Geometry: final body of the model. Coordinates: model frame, mm. Face numbers are marked on the shaded views. A direction names the side the tool comes from. Coordinates: 2 decimals unless noted, no trailing zeros. Order: outer loops, then holes, each group sorted by start corner. A loop starts at its lowest first (then second) coordinate and runs counter-clockwise, first axis right, second up. Notation, with made-up numbers: M 53.5,-8 L 109.5,-8 A15 cw 109.5,13 Z; hole C 77.5,-4 d1. An arc over 180 degrees is marked long. Write item = value, one per line.
from build123d import *

# Parameters (mm, degrees)
F1_DEPTH  = 320
F2_W      = 30
F2_H      = 320
F3_DEPTH  = 428
F5_DEPTH  = 205
F7_W      = 260
F7_H      = 128.6325914682
F8_DEPTH  = 30
F9_W      = 7.5
F9_H      = 457.219858036
F10_DEPTH = 977
F6_W      = 20
F6_H      = 50
F6_H_2    = 25
F11_DEPTH = 25
F12_R     = 5.1978686685
F13_DEPTH = 63


with BuildPart() as f1:
    # F0 (on Front) → F1 (new body)
    with BuildSketch(Plane.XZ):
        with BuildLine():
            Line((150.299176857, 1.1440683747), (180.299176857, 1.1440683747))
            Line((180.299176857, 1.1440683747), (340.299176857, 1.1440683747))
            add(Edge.make_bspline(
                [(340.299176857, 1.1440683747), (349.1569172885, 24.1151609846), (251.1032390966, 88.0444564268), (175.3079980464, 151.1440683747)],
                knots=[0.4586039165, 0.4586039165, 0.4586039165, 0.4586039165, 1, 1, 1, 1], degree=3))
            Line((175.3079980464, 151.1440683747), (145.3079980464, 151.1440683747))
            Line((145.3079980464, 151.1440683747), (0.299176857, 1.1440683747))
            Line((0.299176857, 1.1440683747), (100.299176857, 1.1440683747))
            Line((100.299176857, 1.1440683747), (150.299176857, 1.1440683747))
        make_face()
    extrude(amount=F1_DEPTH)

    # F2 (on face) → F3 (join)
    with BuildSketch(Plane.XY.offset(151.1440683747)):
        with Locations((160.3079980464, -160)):
            Rectangle(F2_W, F2_H)
    extrude(amount=F3_DEPTH)

    # F4 (on face) → F5 (cut)
    with BuildSketch(Plane(origin=(145.3079980464, 0, 0), x_dir=(0, -1, 0), z_dir=(-1, 0, 0))):
        with BuildLine():
            Line((0, 579.1440683747), (0, 151.1440683747))
            add(Edge.make_bspline(
                [(60, 368.6685562134), (50.1739969339, 296.0916949665), (25.086998467, 223.6178816706), (0, 151.1440683747)],
                knots=[0.4913001533, 0.4913001533, 0.4913001533, 0.4913001533, 1, 1, 1, 1], degree=3))
            Line((60, 368.6685562134), (60, 579.1440683747))
            Line((60, 579.1440683747), (0, 579.1440683747))
        make_face()
        with BuildLine():
            add(Edge.make_bspline(
                [(320, 151.1440683747), (294.913001533, 223.6178816706), (269.8260030661, 296.0916949665), (260, 368.6685562134)],
                knots=[0, 0, 0, 0, 0.5086998467, 0.5086998467, 0.5086998467, 0.5086998467], degree=3))
            Line((320, 151.1440683747), (320, 579.1440683747))
            Line((320, 579.1440683747), (260, 579.1440683747))
            Line((260, 579.1440683747), (260, 368.6685562134))
        make_face()
    extrude(amount=-F5_DEPTH, mode=Mode.SUBTRACT)

    # F7 (on face) → F8 (cut)
    with BuildSketch(Plane(origin=(-0.4170581217, 0, 0.4031807106), x_dir=(0, -1, 0), z_dir=(-0.7189672474, 0, 0.6950439534))):
        with Locations((160, 105.3467844897)):
            Rectangle(F7_W, F7_H)
    extrude(amount=-F8_DEPTH, mode=Mode.SUBTRACT)

    # F9 (on face) → F10 (cut)
    with BuildSketch(Plane.XZ.offset(320)):
        with Locations((154.0579980464, 379.7539973927)):
            Rectangle(F9_W, F9_H)
        with Locations((166.5579980464, 379.7539973927)):
            Rectangle(F9_W, F9_H)
    extrude(amount=-F10_DEPTH, mode=Mode.SUBTRACT)

    # F6 (on face) → F11 (join)
    with BuildSketch(Plane.YZ.offset(175.3079980464)):
        with Locations((-250, 554.1440683747)):
            Rectangle(F6_W, F6_H)
        with Locations((-70, 554.1440683747)):
            Rectangle(F6_W, F6_H)
        with Locations((-230, 406.1685562134)):
            Rectangle(F6_W, F6_H_2)
        with Locations((-90, 406.1685562134)):
            Rectangle(F6_W, F6_H_2)
    extrude(amount=-F11_DEPTH)

    # F12 (on Right) → F13 (cut)
    with BuildSketch(Plane.YZ):
        with Locations((-268.3978974819, 7.7915792353)):
            Circle(F12_R)
    extrude(amount=F13_DEPTH, mode=Mode.SUBTRACT)


solid = f1.part
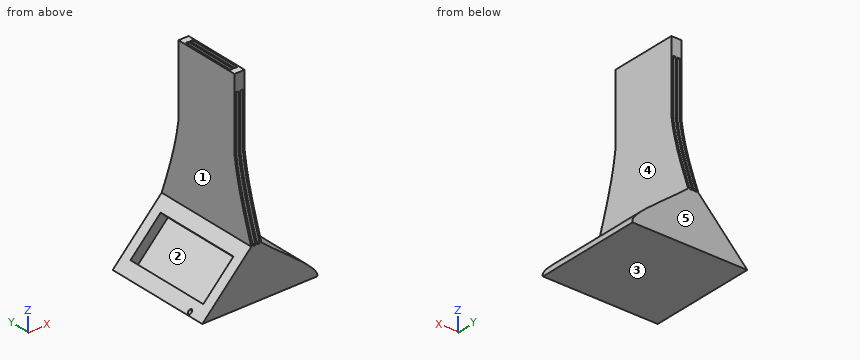
1) Section C-C, the plane y = -231.5. Give the number of separate pieces and of enclosed holes in the cut face, and give its area (3 significant figures).
Numbers:
separate_pieces = 1
enclosed_holes = 2
area = 32,200 mm²
2) Section A-A, the plane z = 539. Return loops of the section in (x, y).
Numbers:
outline = M 145.31,-260 L 175.31,-260 L 175.31,-60 L 145.31,-60 Z; hole M 150.31,-240 L 157.81,-240 L 157.81,-80 L 150.31,-80 Z; hole M 162.81,-240 L 170.31,-240 L 170.31,-80 L 162.81,-80 Z
3) Mould query, pull axis Z, two halves, no side actions, for the marked faces 1, 2 and 3. Classes: pulls with the +Z half, pulls with the -Z half, needs draft (parallel to the pull), parting line crosses it, or undercut.
Numbers:
face_1 = needs draft
face_2 = undercut
face_3 = pulls with the -Z half
4) Pin query (flat end, axial travel): pin 1 (8 mm diameter, centred on x = 156, z = 404, fed in from -Y); pin 2 (5 mm diameter, centred on y = -111, z = 424, fed in from -X); pin 3 (5 mm diameter, centred on y = -135, z = 326.5, fed in from +X). Return the tip coordinate at first contact, or that it passes through.
Numbers:
pin_1 = -260
pin_2 = 145.31
pin_3 = 175.31
5) Section B-B, the plane x = 43. Return loops of the section in (y, z), and give its area (3 significant figures).
Numbers:
outline = M -320,1.14 L 0,1.14 L 0,45.31 L -30,45.31 L -30,15.5 L -290,15.5 L -290,45.31 L -320,45.31 Z; hole C -268.4,7.79 d10.4
area = 6,300 mm²
6) Line query: L1, parallel to X at y = -246, z = 308; L2, parallel to Z at x = 302.5, y = -54; L3, parallel to X at y = -223, z = 396.5. Output: solid intervals per line, ascending.
Numbers:
L1 = 145.31 to 150.31, 157.81 to 162.81, 170.31 to 175.31
L2 = 1.14 to 50.34
L3 = 145.31 to 175.31
7) Set-up query: the marked faces 4 and 5. Return all of +Z, -Z, +X, -X, +Y, -Y with unobstructed straight access to the full face (end or side cutting, diameter ignored); none if empty.
Numbers:
face_4 = +Z, +X, +Y, -Y
face_5 = +Z, -Z, +X, -X, +Y
